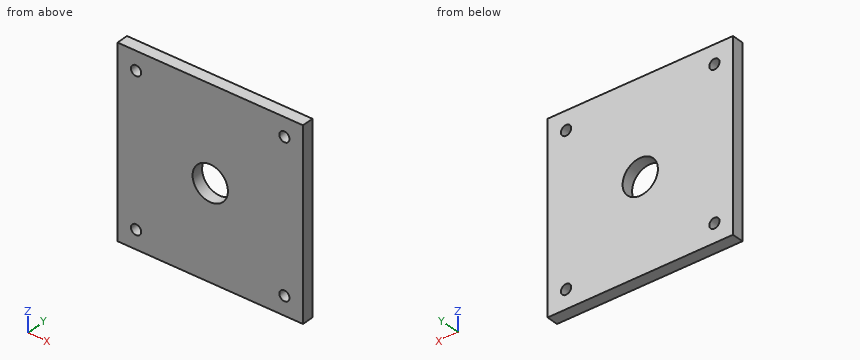
Autodesk Inventor part; units mm, degrees
ref_plane "YZ Plane" through (0, 0, 0) normal (1, 0, 0) x (0, 1, 0)
ref_plane "XZ Plane" through (0, 0, 0) normal (0, 1, 0) x (-1, 0, 0)
ref_plane "XY Plane" through (0, 0, 0) normal (0, 0, 1) x (1, 0, 0)
sketch "Sketch1" plane through (0, 0, 0) normal (0, 1, 0) x (-1, 0, 0)
  line L0 (50, 50) -> (-50, 50)
  line L1 (-50, 50) -> (-50, -50)
  line L2 (-50, -50) -> (50, -50)
  line L3 (50, -50) -> (50, 50)
  line L4 (50, 50) -> (-50, -50) construction
  line L5 (-50, 50) -> (50, -50) construction
  point P0 (0, 0)
  dimension "d0" = 100
  dimension "d1" = 100
extrude "Extrusion1" add sketch "Sketch1" along normal blind 6.35
sketch "Sketch2" plane through (0, 6.35, 0) normal (0, 1, 0) x (1, 0, 0)
  line L0 (40, -40) -> (-40, -40) construction
  line L1 (-40, -40) -> (-40, 40) construction
  line L2 (-40, 40) -> (40, 40) construction
  line L3 (40, 40) -> (40, -40) construction
  line L4 (40, -40) -> (-40, 40) construction
  line L5 (-40, -40) -> (40, 40) construction
  line L6 (-50, -50) -> (50, -50)
  line L7 (50, -50) -> (50, 50)
  line L8 (50, 50) -> (-50, 50)
  line L9 (-50, 50) -> (-50, -50)
  point P0 (0, 0)
  dimension "d4" = 80
  dimension "d5" = 80
  dimension "d20" = 100
hole "Hole1" at (-40, 6.35, 40) at (-40, 6.35, -40) at (40, 6.35, -40) at (40, 6.35, 40) direction (0, -1, 0) diameter 5.5 depth 8 tip angle 118
sketch "Sketch3" plane through (0, 6.35, 0) normal (0, 1, 0) x (1, 0, 0)
  point P0 (0, 0)
  point P1 (0, 0)
hole "Hole2" at (0, 6.35, 0) direction (0, -1, 0) diameter 19.05 end through all
equation "\"d5\" = d4"
properties part number "topPlate"
Could you check a few things on this model? Use its own coordinates, in mm. Give positions to 0.01 mm unless a question says otherwise; leave off trailing zeros. Order: outer loops, then holes, each group sorted by start corner. A loop starts at its lowest first (then second) coordinate and runs counter-clockwise, first axis right, second up. Notation, with made-up numbers: (5.5, 51.5) - (28.5, 51.5) arc R3 ccw to (28.5, 56.5) - close; hole circle Ø7 at (7.5, 48.5). An arc over 180 degrees is marked (long way). One line per item, written item: value. Start each with the question number.
1. Imagine slicing it at B-B on z = 0. List the corners of the cut face in (x, y) for me (3 decimals), plus the area to 3 significant figures.
2. If I drill on probe 1 along Z at (x, y) = (-40, 4.25); probe 2 along X at (y, z) = (5, 0) (3 decimals), over which ranges is the centre line in solid material (lowest first)?
3. Imagine slicing it at C-C on y = 3.75. List the corners of the cut face in (x, z) for me (3 decimals), plus the area to 3 significant figures.
4. Imagine slicing it at A-A on z = -40. List the corners of the cut face in (x, y) for me, plus the area to 3 significant figures.
5. Imagine slicing it at D-D on x = -1.5. List the corners of the cut face in (y, z) for me.
Values:
1. outline: (-50, 0) - (-9.525, 0) - (-9.525, 6.35) - (-50, 6.35) - close; (9.525, 0) - (50, 0) - (50, 6.35) - (9.525, 6.35) - close
1. area: 514 mm²
2. probe 1: -50 to -42.75, -37.25 to 37.25, 42.75 to 50
2. probe 2: -50 to -9.525, 9.525 to 50
3. outline: (-50, -50) - (50, -50) - (50, 50) - (-50, 50) - close; hole circle Ø5.5 at (-40, -40); hole circle Ø5.5 at (-40, 40); hole circle Ø19.05 at (0, 0); hole circle Ø5.5 at (40, -40); hole circle Ø5.5 at (40, 40)
3. area: 9,620 mm²
4. outline: (-50, 0) - (-42.75, 0) - (-42.75, 6.35) - (-50, 6.35) - close; (-37.25, 0) - (37.25, 0) - (37.25, 6.35) - (-37.25, 6.35) - close; (42.75, 0) - (50, 0) - (50, 6.35) - (42.75, 6.35) - close
4. area: 565 mm²
5. outline: (0, -50) - (6.35, -50) - (6.35, -9.41) - (0, -9.41) - close; (0, 9.41) - (6.35, 9.41) - (6.35, 50) - (0, 50) - close
